Could you check a few things on this model? Use its own coordinates, in mm. A direction names the side the tool comes from. Coordinates: 2 decimals unless noted, no trailing zeros. Write each loop counter-clockwise with the first axis right and the second up, starting at its lowest first coordinate (ties: lowest second). Pieces come first, ordered by that corner, then holes. Notation, with made-up numbers: (-5, -31) - (8, -31) arc R21 ccw to (8, -22) - close; hole circle Ø3 at (42, 87). An arc over 180 degrees is marked (long way). Answer as a JSON object with one key per item and string values. Group by question number.
1) Please list where these lines run through material, in increasing order: line 1 along Z through (x, y) = (0, 0); line 2 along X through (y, z) = (-2.75, -2.5); line 3 along X through (y, z) = (2.25, 4).
2) If we section it at C-C (y = -5): Write out the boundary of the cut face in (x, z), plus the area to 3 significant figures.
3) If we section it at B-B (x = -0.5): Write out the boundary of the cut face in (y, z).
4) On a 3-axis mill with a long thin cutter (end or side, diameter ignored), from which of +Z, -Z, +X, -X, +Y, -Y can I reach the whole of each face in a straight line? I mean faces 4 (the flat face through (6, 0, 3)), 5 (the flat face through (8.859, -6.884, 0.947)). Say none if no direction works.
5) We'd pull the mould along Z, two halves only. Please class faces 1 (the flat face through (6, -2.5, 0)), 2 (the flat face through (8.904, -6.884, -0.921)), 3 (the flat face through (-0.947, -6.884, 8.859)): released by +Z, released by -Z, zero draft, split by the parting line, or undercut.
6) Will these pins go through, and if not, where does the flat tip stop? pin 1 Ø0.8 at (x, z) = (-6.5, 1) entering from +Y; pin 2 Ø1.5 at (x, y) = (-7.5, -1) entering from -Z; pin 3 Ø3.5 at (x, z) = (0, 0) entering from +Y.
7) If we section it at A-A (y = -1.25): Write out the boundary of the cut face in (x, z), plus the area to 3 significant figures.
```python
from build123d import *

# Parameters (mm, degrees)
SKETCH9_R           = 7.5
BOSS_EXTRUDE2_DEPTH = 7.5
SKETCH10_W          = 17.888516884
SKETCH10_H          = 18.524036688
CUT_EXTRUDE2_DEPTH  = 20
SKETCH15_W          = 6
SKETCH15_H          = 5
CUT_EXTRUDE3_DEPTH  = 20
BOSS_EXTRUDE4_DEPTH = 1.25
SKETCH24_R          = 1.5
CUT_EXTRUDE4_DEPTH  = 15
BOSS_EXTRUDE5_DEPTH = 1.25


with BuildPart() as part:
    # Sketch7 → Revolve1 (revolve)
    with BuildSketch(Plane(origin=(0, 0, 0), x_dir=(1, 0, 0), z_dir=(0, 1, 0))):
        with BuildLine():
            Line((7.5, 0), (6.25, 0))
            ThreePointArc((6.25, 0), (0, -6.25), (-6.25, 0))
            Line((-6.25, 0), (-7.5, 0))
            ThreePointArc((-7.5, 0), (0, -7.5), (7.5, 0))
        make_face()
    revolve(axis=Axis((-6.25, 0, 0), (-1, 0, 0)))

    # Sketch10 → Cut-Extrude2 (cut)
    with BuildSketch(Plane(origin=(0, 2.5, 0), x_dir=(-1, 0, 0), z_dir=(0, -1, 0))):
        with Locations((-0.350209641, -0.603260139)):
            Rectangle(SKETCH10_W, SKETCH10_H)
    extrude(amount=-CUT_EXTRUDE2_DEPTH, mode=Mode.SUBTRACT)


with BuildPart() as body_2:
    # Sketch9 → Boss-Extrude2 (new body)
    with BuildSketch(Plane(origin=(0, 0, 0), x_dir=(1, 0, 0), z_dir=(0, 1, 0))):
        with Locations(Location((0, 0, 0), (0, 0, 270))):
            Circle(SKETCH9_R)
    extrude(amount=-BOSS_EXTRUDE2_DEPTH)

    # Sketch12 → Cut-Revolve4 (revolve, cut)
    with BuildSketch(Plane(origin=(0, 0, 0), x_dir=(1, 0, 0), z_dir=(0, 1, 0))):
        with BuildLine():
            Line((-6.75, 0), (6.75, 0))
            ThreePointArc((6.75, 0), (0, 6.75), (-6.75, 0))
        make_face()
    revolve(axis=Axis((-8.960272056, 0, 0), (1, 0, 0)), mode=Mode.SUBTRACT)


with BuildPart() as cut_extrude3_tool:
    # Sketch15 → Cut-Extrude3 (new body)
    with BuildSketch(Plane(origin=(7.5, 0, 0), x_dir=(0, 0, -1), z_dir=(1, 0, 0))):
        Rectangle(SKETCH15_W, SKETCH15_H)
    extrude(amount=-CUT_EXTRUDE3_DEPTH)


with BuildPart() as part_1:
    add(part.part)

    # Cut-Extrude3: cut by cut_extrude3_tool
    add(cut_extrude3_tool.part, mode=Mode.SUBTRACT)


with BuildPart() as body_2_1:
    add(body_2.part)

    # Cut-Extrude3: cut by cut_extrude3_tool
    add(cut_extrude3_tool.part, mode=Mode.SUBTRACT)

    # Sketch23 → Boss-Extrude4 (add)
    with BuildSketch(Plane.XZ.offset(7.5)):
        with BuildLine():
            Line((-10.5, 0), (-7.263493829, -1.868597709))
            ThreePointArc((-7.263493829, -1.868597709), (-7.5, 0), (-7.263493829, 1.868597709))
            Line((-7.263493829, 1.868597709), (-10.5, 0))
        make_face()
    boss_extrude4 = extrude(amount=-BOSS_EXTRUDE4_DEPTH)

    # Mirror1: Boss-Extrude4 across plane
    add(boss_extrude4.mirror(Plane(origin=(0, 0, 0), x_dir=(0, 0, 1), z_dir=(1, 0, 0))))


with BuildPart() as cut_extrude4_tool:
    # Sketch24 → Cut-Extrude4 (new body)
    with BuildSketch(Plane.XZ.offset(7.5)):
        with Locations(Location((0, 0, 0), (0, 0, 90))):
            Circle(SKETCH24_R)
    extrude(amount=-CUT_EXTRUDE4_DEPTH)


with BuildPart() as part_2:
    add(part_1.part)

    # Cut-Extrude4: cut by cut_extrude4_tool
    add(cut_extrude4_tool.part, mode=Mode.SUBTRACT)



with BuildPart() as body_2_2:
    add(body_2_1.part)

    # Cut-Extrude4: cut by cut_extrude4_tool
    add(cut_extrude4_tool.part, mode=Mode.SUBTRACT)


with BuildPart() as part_3:
    add(part_2.part)

    add(body_2_2.part)  # Boss-Extrude5 merges body 2
    # Sketch25 → Boss-Extrude5 (add)
    with BuildSketch(Plane.XZ.offset(7.5)):
        with BuildLine():
            Line((0, 10.5), (1.868597709, 7.263493829))
            ThreePointArc((1.868597709, 7.263493829), (0, 7.5), (-1.868597709, 7.263493829))
            Line((-1.868597709, 7.263493829), (0, 10.5))
        make_face()
    boss_extrude5 = extrude(amount=-BOSS_EXTRUDE5_DEPTH)

    # Mirror2: Boss-Extrude5 across plane
    add(boss_extrude5.mirror(Plane.XY))


solid = part_3.part
```
Here are the results:
{
 "1": {"line 1": "z = -7.5 to -6.25, 6.25 to 7.5", "line 2": "x = -7.07 to -5.02, 5.02 to 7.07", "line 3": "x = -5.93 to -4.24, 4.24 to 5.93"},
 "2": {"outline": "circle Ø15 at (0, 0); hole circle Ø7.5 at (0, 0)", "area": "133 mm²"},
 "3": {"outline": "(-7.5, -9.63) - (-6.25, -9.63) - (-6.25, -7.48) - (0, -7.48) arc R7.48 ccw to (2.5, -7.05) - (2.5, -5.71) arc R6.23 cw to (-6.07, -1.41) - (-7.5, -1.41) - close; (-7.5, 1.41) - (-6.07, 1.41) arc R6.23 cw to (2.5, 5.71) - (2.5, 7.05) arc R7.48 ccw to (0, 7.48) - (-6.25, 7.48) - (-6.25, 9.63) - (-7.5, 9.63) - close"},
 "4": {"face 4": "+X, -X, +Y", "face 5": "+Z, +X, +Y, -Y"},
 "5": {"face 1": "undercut", "face 2": "released by -Z", "face 3": "released by +Z"},
 "6": {"pin 1": "stops at y = -2.5", "pin 2": "stops at z = -3.27", "pin 3": "stops at y = -6"},
 "7": {"outline": "(-6.87, -3) arc R7.5 ccw to (6.87, -3) - (5.34, -3) arc R6.12 cw to (-5.34, -3) - close; (-6.87, 3) - (-5.34, 3) arc R6.12 cw to (5.34, 3) - (6.87, 3) arc R7.5 ccw to start", "area": "41.8 mm²"}
}
